Could you check a few things on this model? Use its own coordinates, in mm. Face numbers are marked on the shaded views. A direction names the side the tool comes from. Give positions to 0.01 mm unless a question says otherwise; leave off trailing zeros. Order: outer loops, then holes, each group sorted by start corner. A loop starts at its lowest first (then second) coordinate and runs counter-clockwise, first axis right, second up.
(1) Imagine slicing it at A-A, the plane y = -8. Write out the boundary of the cut face in (x, z), then the cut area to 4 significant figures.
(2) Imagine slicing it at B-B, the plane x = -3. Write out the boundary of the cut face in (y, z), then the cut area to 3 significant figures.
(3) If I drill on probe 1 along Z at (x, y) = (-13.75, -3.5); probe 2 along Y at (x, z) = (-12.25, 10.5); probe 3 along Y at (x, z) = (-2, 11), over which ranges is the centre line in solid material (lowest first)?
(4) Imagine slicing it at C-C, the plane x = 2.75. Write out the boundary of the cut face in (y, z).
(5) Will these pins go through, and if not, where does the flat tip stop? pin 1 (10 mm diameter, centred on x = -10, z = 12, fed in from -Y); pin 2 (6 mm diameter, centred on x = -13.5, y = -7, fed in from -Z); pin 3 (4 mm diameter, centred on x = -14.5, y = -7, fed in from -Z).
(6) On a 3-axis mill with a long thin cutter (end or side, diameter ignored), from which of +Z, -Z, +X, -X, +Y, -Y can I reach the whole of each face in a straight line? I mean the marked faces 5, 6 and 7. Say none if no direction works.
(7) Imagine slicing it at D-D, the plane z = 9.5. Write out the boundary of the cut face in (x, y), then the cut area to 3 significant figures.
(8) If we mould it in two halves opening along Y, with no side actions, what happens to the marked faces 1, 2, 3 and 4? For each: released by +Y, released by -Y, zero draft, split by the parting line, or undercut.
from build123d import *

# Parameters (mm, degrees)
SALIENTE_EXTRUIR1_DEPTH = 18
REDONDEO1_R             = 17
CROQUIS5_W              = 36
CROQUIS5_H              = 3
SALIENTE_EXTRUIR4_DEPTH = 15
CROQUIS6_W              = 15
CROQUIS6_H              = 2.25
SALIENTE_EXTRUIR5_DEPTH = 10
CROQUIS7_W              = 15
CROQUIS7_H              = 2.25
SALIENTE_EXTRUIR6_DEPTH = 10
SALIENTE_EXTRUIR7_REACH = 53.008
CROQUIS9_W              = 14.804118301
CROQUIS9_H              = 37.418244965
CORTAR_EXTRUIR1_DEPTH   = 65.529262729
CORTAR_EXTRUIR2_DEPTH   = 43.150382534
CROQUIS13_W             = 6.782058138
CROQUIS13_H             = 38.050659694
CORTAR_EXTRUIR4_DEPTH   = 66.385361662
CORTAR_EXTRUIR5_DEPTH   = 59.680118278
CROQUIS15_R             = 67.5
CORTAR_EXTRUIR6_DEPTH   = 53.753520742


with BuildPart() as part:
    # Croquis1 → Saliente-Extruir1 (new, symmetric)
    with BuildSketch(Plane.XY):
        Polygon((-23.009210442, -16.267830887), (-23.009210442, 0), (5.722840366, 49.765371804), (7.454891173, 46.765371804), (-20.009210442, -0.803847577), (-20.009210442, -16.267830887), align=None)
    extrude(amount=SALIENTE_EXTRUIR1_DEPTH, both=True)

    # Redondeo1
    redondeo1_edges = [part.edges().sort_by_distance(p)[0] for p in [
        (-23.009210442, 0, 0),
    ]]
    fillet(redondeo1_edges, radius=REDONDEO1_R)

    # Croquis8 → Saliente-Extruir7 (add, up to next)
    with BuildSketch(Plane(origin=(-7.962730425, 4.597284555, 0), x_dir=(0, 0, 1), z_dir=(-0.8660254037844399, 0.49999999999999806, 0)), mode=Mode.PRIVATE) as saliente_extruir7_sk1:
        Polygon((18, -14.092960033), (18, -1.092960033), (15.75, -1.092960033), (15.75, -11.092960033), (7.5, -11.092960033), (7.5, -1.092960033), (5.25, -1.092960033), (5.25, -11.092960033), (-18, -11.092960033), (-18, -14.092960033), align=None)
    saliente_extruir7_tool1 = extrude(saliente_extruir7_sk1.sketch, amount=SALIENTE_EXTRUIR7_REACH, mode=Mode.PRIVATE) - part.part


with BuildPart() as body_2:
    # Croquis5 → Saliente-Extruir4 (new body)
    with BuildSketch(Plane(origin=(-7.962730425, 4.597284555, 0), x_dir=(0, 0, -1), z_dir=(0.8660254037844398, -0.499999999999998, 0))):
        with Locations((0, -12.592960033)):
            Rectangle(CROQUIS5_W, CROQUIS5_H)
    extrude(amount=SALIENTE_EXTRUIR4_DEPTH)

    # Croquis6 → Saliente-Extruir5 (add)
    with BuildSketch(Plane(origin=(-5.546480017, -9.606785192, 0), x_dir=(0.8660254037844398, -0.49999999999999806, 0), z_dir=(0.499999999999998, 0.8660254037844397, 0))):
        with Locations((-1.694569109, -16.875)):
            Rectangle(CROQUIS6_W, CROQUIS6_H)
    extrude(amount=SALIENTE_EXTRUIR5_DEPTH)

    # Croquis7 → Saliente-Extruir6 (add)
    with BuildSketch(Plane(origin=(-5.546480017, -9.606785192, 0), x_dir=(0.8660254037844398, -0.49999999999999806, 0), z_dir=(0.499999999999998, 0.8660254037844397, 0))):
        with Locations((-1.694569109, -6.375)):
            Rectangle(CROQUIS7_W, CROQUIS7_H)
    extrude(amount=SALIENTE_EXTRUIR6_DEPTH)


with BuildPart() as part_1:
    add(part.part)

    add(body_2.part)  # Saliente-Extruir7 merges body 2
    add(saliente_extruir7_tool1.solids().sort_by_distance((-11.75921, -1.978412, 17.617247))[0])

    # Croquis9 → Cortar-Extruir1 (cut, through all)
    with BuildSketch(Plane(origin=(0, 41.27, 0), x_dir=(1, 0, 0), z_dir=(0, 1, 0))):
        with Locations((0.741451059, 0.142817729)):
            Rectangle(CROQUIS9_W, CROQUIS9_H)
    extrude(amount=CORTAR_EXTRUIR1_DEPTH, mode=Mode.SUBTRACT)

    # Croquis11 → Cortar-Extruir2 (cut, through all)
    with BuildSketch(Plane(origin=(-17.256907831, 9.963280382, 0), x_dir=(0, 0, 1), z_dir=(-0.8660254037844386, 0.5000000000000003, 0))):
        Polygon((8.788629382, 36.149885998), (18, 36.149885998), (18, 23.351498504), align=None)
    extrude(amount=-CORTAR_EXTRUIR2_DEPTH, mode=Mode.SUBTRACT)

    # Croquis13 → Cortar-Extruir4 (cut, through all)
    with BuildSketch(Plane(origin=(18.074942999, 31.306719618, 0), x_dir=(-0.8660254037844386, 0.4999999999999999, 0), z_dir=(-0.49999999999999994, -0.8660254037844387, 0))):
        with Locations((17.8722453, 0.046357502)):
            Rectangle(CROQUIS13_W, CROQUIS13_H)
    extrude(amount=-CORTAR_EXTRUIR4_DEPTH, mode=Mode.SUBTRACT)

    # Croquis14 → Cortar-Extruir5 (cut, through all)
    with BuildSketch(Plane(origin=(7.886305076, 13.659481075, 21.914651455), x_dir=(0.9563939122686984, -0.15449956154835387, -0.24787208406099226), z_dir=(0.29207992840209546, 0.5058972758635086, 0.8116386275298311))):
        Polygon((-2.921520295, 29.452632093), (-8.700629296, 32.1607213), (-16.69781327, 15.094592988), (-10.918704269, 12.386503781), align=None)
    extrude(amount=CORTAR_EXTRUIR5_DEPTH, mode=Mode.SUBTRACT)

    # Croquis15 → Cortar-Extruir6 (cut, through all)
    with BuildSketch(Plane.ZY.offset(23.009210442)):
        with Locations((-57.422816505, -44.474628196)):
            Circle(CROQUIS15_R)
    extrude(amount=-CORTAR_EXTRUIR6_DEPTH, mode=Mode.SUBTRACT)


solid = part_1.part
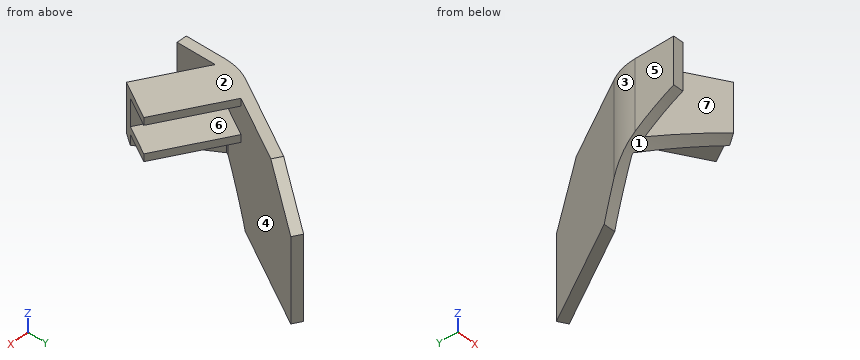
Answer block:
1. outline: (-23.01, -0.63) - (-20.01, -0.63) - (-20.01, 18) - (-23.01, 18) - close; (-14.33, -0.63) - (-8.33, -0.63) - (-8.33, 5.25) - (2.08, 5.25) - (2.08, 7.5) - (-8.33, 7.5) - (-8.33, 15.75) - (2.08, 15.75) - (2.08, 18) - (-14.33, 18) - close
1. area: 214.5 mm2
2. outline: (-14.54, 3.08) arc R67.5 cw to (-11.08, 1.24) - (-11.08, 5.25) - (0.47, 5.25) - (0.47, 7.5) - (-11.08, 7.5) - (-11.08, 15.75) - (0.47, 15.75) - (0.47, 18) - (-14.54, 18) - close; (28.66, -18) - (34.66, -18) - (34.66, 12.74) - (28.66, 16.48) - close
2. area: 302 mm2
3. probe 1: z = 5.25 to 7.5, 15.75 to 18
3. probe 2: y = -9.2 to -5.74, 12.64 to 18.64
3. probe 3: y = -15.07 to -11.65, 30.39 to 36.39
4. outline: (-6.85, 5.25) - (-2.85, 5.25) - (-2.85, 7.5) - (-6.85, 7.5) - close; (-6.85, 15.75) - (-2.85, 15.75) - (-2.85, 18) - (-6.85, 18) - close; (38.62, -18) - (40.15, -18) - (40.15, 7.25) - (38.62, 8.21) - close
5. pin 1: stops at y = -13.39
5. pin 2: stops at z = -3.19
5. pin 3: stops at z = -2.67
6. face 5: +Z, -Z, -X, +Y, -Y
6. face 6: +X
6. face 7: +Z, -Z, -Y
7. outline: (-23.01, -16.27) - (-20.01, -16.27) - (-20.01, -4.72) - (-2.02, -15.11) - (-0.52, -12.51) - (-20.01, -1.26) - (-20.01, -0.8) - (1.85, 37.06) - (-0.75, 38.56) - (-20.73, 3.94) arc R17 ccw to (-23.01, -4.56) - close
7. area: 243 mm2
8. face 1: released by -Y
8. face 2: zero draft
8. face 3: released by +Y
8. face 4: undercut
